Can you work these out from the model? Positions are in its coordinate system, mm. Round coordinates to 2 decimals unless told otherwise and drop trailing zeros. Loops run counter-clockwise (first coordinate to the right, second up) from the corner with the lowest first, then second, coordinate; pieces in that order, holes last.
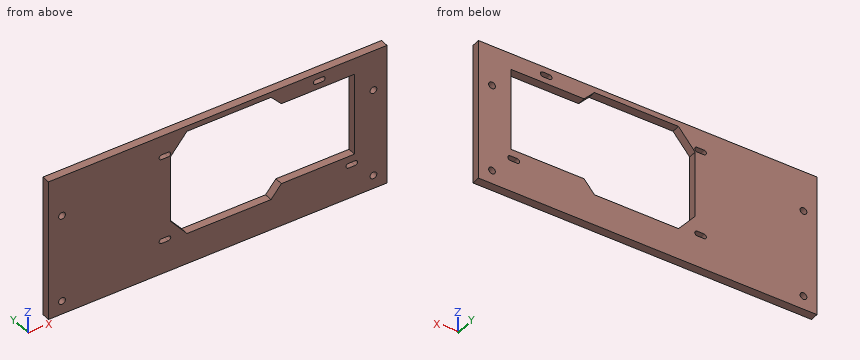
```python
from build123d import *

# Parameters (mm, degrees)
SKETCH1_W           = 250
SKETCH1_H           = 105
BOSS_EXTRUDE1_DEPTH = 6
SKETCH1_4_R         = 2.5
CUT_EXTRUDE1_DEPTH  = 6


with BuildPart() as part:
    # Sketch1 → Boss-Extrude1 (new body)
    with BuildSketch(Plane(origin=(0, 0, 0), x_dir=(1, 0, 0), z_dir=(0, 1, 0))):
        Rectangle(SKETCH1_W, SKETCH1_H)
    extrude(amount=BOSS_EXTRUDE1_DEPTH)

    # Sketch1<4> → Cut-Extrude1 (cut)
    with BuildSketch(Plane(origin=(0, 0, 0), x_dir=(1, 0, 0), z_dir=(0, 1, 0))):
        with Locations((-115, -22.5)):
            Circle(SKETCH1_4_R)
        with Locations((-115, 42.5)):
            Circle(SKETCH1_4_R)
        with Locations((115, 42.5)):
            Circle(SKETCH1_4_R)
        with Locations((115, -22.5)):
            Circle(SKETCH1_4_R)
        Polygon((-22.728448276, 29.5), (39.383174792, 29.5), (47, 20.5), (101, 20.5), (101, -40.5), (47, -40.5), (39.383174792, -48.5), (-22.728448276, -48.5), (-35, -34), (-35, 15), align=None)
        with BuildLine():
            Line((72.5, -44.7), (77.5, -44.7))
            ThreePointArc((77.5, -44.7), (79.3, -46.5), (77.5, -48.3))
            Line((77.5, -48.3), (72.5, -48.3))
            ThreePointArc((72.5, -48.3), (70.7, -46.5), (72.5, -44.7))
        make_face()
        with BuildLine():
            Line((96.5, 29.3), (101.5, 29.3))
            ThreePointArc((101.5, 29.3), (103.3, 27.5), (101.5, 25.7))
            Line((101.5, 25.7), (96.5, 25.7))
            ThreePointArc((96.5, 25.7), (94.7, 27.5), (96.5, 29.3))
        make_face()
        with BuildLine():
            Line((-41.5, 29.3), (-36.5, 29.3))
            ThreePointArc((-36.5, 29.3), (-34.7, 27.5), (-36.5, 25.7))
            Line((-36.5, 25.7), (-41.5, 25.7))
            ThreePointArc((-41.5, 25.7), (-43.3, 27.5), (-41.5, 29.3))
        make_face()
        with BuildLine():
            Line((-41.5, -34.7), (-36.5, -34.7))
            ThreePointArc((-36.5, -34.7), (-34.7, -36.5), (-36.5, -38.3))
            Line((-36.5, -38.3), (-41.5, -38.3))
            ThreePointArc((-41.5, -38.3), (-43.3, -36.5), (-41.5, -34.7))
        make_face()
    extrude(amount=CUT_EXTRUDE1_DEPTH, mode=Mode.SUBTRACT)


solid = part.part
```
(1) Suppose I cut it at A-A (z = -42.5). Write out the boundary of the cut face in (x, y), then the cut area to 3 significant figures.
(2) Suppose I cut it at C-C (z = -6.5). Write out the boundary of the cut face in (x, y).
(3) Suppose I cut it at B-B (x = 115). Write out the boundary of the cut face in (y, z).
(4) If I drill on line 1 (Z direction, x = 115, y = 1.7); line 2 (Z direction, x = 74, y = 5.3); line 3 (X direction, y = 3.5, z = 22.5), over which ranges is the centre line in solid material (lowest first)?
(5) Suppose I cut it at D-D (y = 4.75). Give the number of separate pieces and of enclosed holes in the cut face, then the cut area to 3 significant figures.
Check result:
1. outline: (-125, 0) - (-117.5, 0) - (-117.5, 6) - (-125, 6) - close; (-112.5, 0) - (112.5, 0) - (112.5, 6) - (-112.5, 6) - close; (117.5, 0) - (125, 0) - (125, 6) - (117.5, 6) - close
1. area: 1,440 mm2
2. outline: (-125, 0) - (-35, 0) - (-35, 6) - (-125, 6) - close; (101, 0) - (125, 0) - (125, 6) - (101, 6) - close
3. outline: (0, -52.5) - (6, -52.5) - (6, -45) - (0, -45) - close; (0, -40) - (6, -40) - (6, 20) - (0, 20) - close; (0, 25) - (6, 25) - (6, 52.5) - (0, 52.5) - close
4. line 1: z = -52.5 to -45, -40 to 20, 25 to 52.5
4. line 2: z = -52.5 to -20.5, 40.5 to 44.7, 48.3 to 52.5
4. line 3: x = -125 to -117.5, -112.5 to -35, 101 to 112.5, 117.5 to 125
5. separate pieces: 1
5. enclosed holes: 9
5. area: 16,600 mm2
